Geometry: see drawing. Coordinates: mm, zero at the bounding-box minimum. Round coordinates to 2 decimals unless told otherwise and drop trailing zeros. Loops run counter-clockwise (first coordinate to the right, second up) from the corner with the lowest first, then second, coordinate; pieces in that order, holes last.
(1) Section C-C, the plane z = 51. Return the cut outline in (x, y) (3 decimals).
(2) First-contact query: pin 1 Ø1 at (y, z) = (1.5, 9) entering from +X; pin 2 Ø1.6 at (y, z) = (2, 186) entering from -X; pin 3 Ø2 at (x, z) = (252.5, 252.5) entering from -Y; pin 4 Ø1 at (y, z) = (2, 104) entering from +X. Flat tips, straight axial feed; report the tip coordinate or a pass-through.
(3) Section B-B, the plane y = 1.4. Count the separate pieces of the cut face and the enclosed holes in it, plus the area to 3 significant figures.
(4) Material intervals for probe 1 along Z at (x, y) = (252.5, 1.1); probe 2 along X at (y, z) = (1.95, 97.5), sorted ascending.
(5) Section A-A, the plane x = 94. Return the cut outline in (y, z) (3 decimals), plus the area to 3 significant figures.
(6) Section D-D, the plane x = 234. Return the cut outline in (y, z) (3 decimals), plus the area to 3 significant figures.
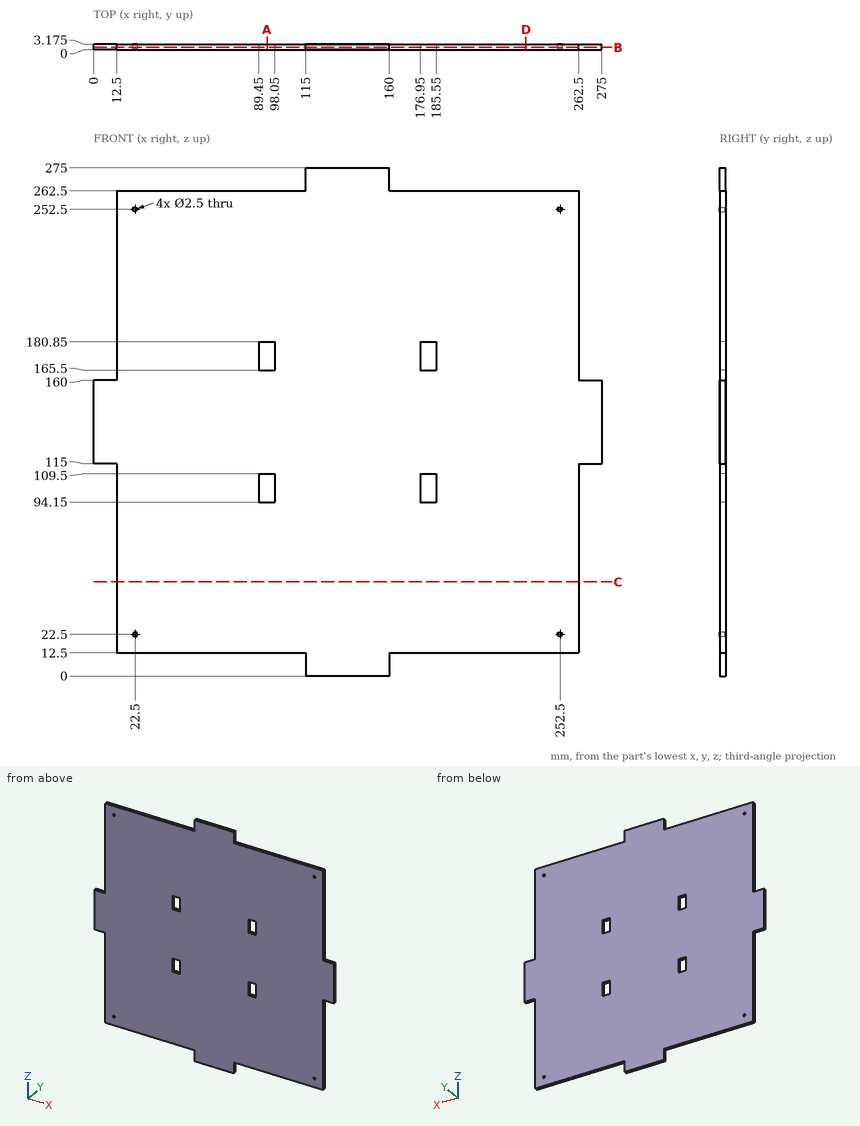
Output values:
1. outline: (12.5, 0) - (262.5, 0) - (262.5, 3.175) - (12.5, 3.175) - close
2. pin 1: stops at x = 160
2. pin 2: stops at x = 12.5
2. pin 3: passes through
2. pin 4: stops at x = 262.5
3. separate pieces: 1
3. enclosed holes: 8
3. area: 64,200 mm2
4. probe 1: z = 12.5 to 21.25, 23.75 to 251.25, 253.75 to 262.5
4. probe 2: x = 12.5 to 89.45, 98.05 to 176.95, 185.55 to 262.5
5. outline: (0, 12.5) - (3.175, 12.5) - (3.175, 94.15) - (0, 94.15) - close; (0, 109.5) - (3.175, 109.5) - (3.175, 165.5) - (0, 165.5) - close; (0, 180.85) - (3.175, 180.85) - (3.175, 262.5) - (0, 262.5) - close
5. area: 696 mm2
6. outline: (0, 12.5) - (3.175, 12.5) - (3.175, 262.5) - (0, 262.5) - close
6. area: 794 mm2
